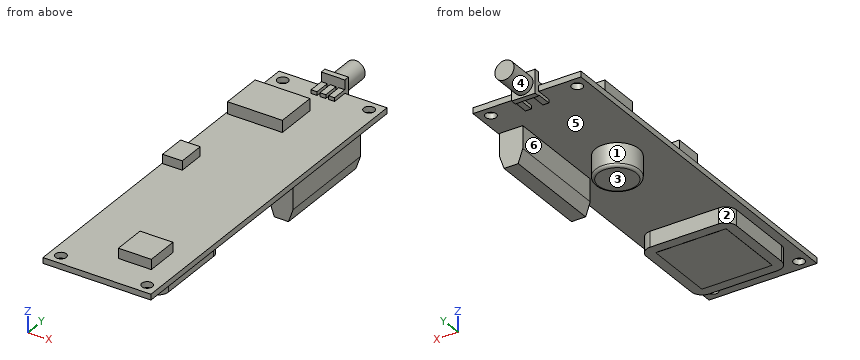
```python
from build123d import *

# Parameters (mm, degrees)
SKETCH3_W            = 1.6002
SKETCH3_H            = 100
BOSS_EXTRUDE1_DEPTH  = 30
SKETCH5_R            = 1.5
SCREW_HOLES_DEPTH    = 13.39
SKETCH7_W            = 6.477
SKETCH7_H            = 28.575
BOSS_EXTRUDE2_DEPTH  = 9.906
CUT_EXTRUDE1_REACH   = 91.18
SKETCH9_R            = 6.0325
BOSS_EXTRUDE3_DEPTH  = 6.35
FILLET1_R            = 0.762
SKETCH10_W           = 25.0698
SKETCH10_H           = 25.0698
BOSS_EXTRUDE4_DEPTH  = 4.318
FILLET2_R            = 3.048
SKETCH11_W           = 19.558
SKETCH11_H           = 19.558
STICKER_DEPTH        = 0.0254
SKETCH12_W           = 15.24
SKETCH12_H           = 11.684
BIG_CHIP_DEPTH       = 3.302
SKETCH13_W           = 9.144
SKETCH13_H           = 9.144
UBLOX_CHIP_DEPTH     = 2.794
SKETCH14_W           = 6.5278
SKETCH14_H           = 6.5278
BOSS_EXTRUDE8_DEPTH  = 1.524
SKETCH15_R           = 2.667
BOSS_EXTRUDE9_DEPTH  = 8.001
SKETCH17_W           = 1.651
SKETCH17_H           = 1.016
BOSS_EXTRUDE10_DEPTH = 4.318
SKETCH18_W           = 1.651
SKETCH18_H           = 0.9652
BOSS_EXTRUDE11_DEPTH = 4.318
SKETCH19_W           = 5.461
SKETCH19_H           = 7.62
USB_CONNECTOR_DEPTH  = 2.54


with BuildPart() as part:
    # Sketch3 → Boss-Extrude1 (new body)
    with BuildSketch(Plane(origin=(0, 0, 0), x_dir=(0, 0, -1), z_dir=(1, 0, 0))):
        with Locations((-0.8001, -50)):
            Rectangle(SKETCH3_W, SKETCH3_H)
    extrude(amount=BOSS_EXTRUDE1_DEPTH)

    # Sketch5 → Screw-Holes (cut)
    with BuildSketch(Plane.XY.offset(1.6002)):
        with Locations((27, -3)):
            Circle(SKETCH5_R)
        with Locations((3, -3)):
            Circle(SKETCH5_R)
        with Locations((3, -97)):
            Circle(SKETCH5_R)
        with Locations((27, -97)):
            Circle(SKETCH5_R)
    extrude(amount=-SCREW_HOLES_DEPTH, mode=Mode.SUBTRACT)

    # Sketch7 → Boss-Extrude2 (add)
    with BuildSketch(Plane(origin=(0, 0, 0), x_dir=(-1, 0, 0), z_dir=(0, 0, -1))):
        with Locations((-26.5075, -25.1079)):
            Rectangle(SKETCH7_W, SKETCH7_H)
    extrude(amount=BOSS_EXTRUDE2_DEPTH)

    # Sketch8 → Cut-Extrude1 (cut, up to next)
    with BuildSketch(Plane(origin=(0, -10.8204, 0), x_dir=(1, 0, 0), z_dir=(0, 1, 0)), mode=Mode.PRIVATE) as cut_extrude1_sk1:
        Polygon((28.476, 9.906), (29.746, 6.223), (29.746, 9.906), align=None)
    cut_extrude1_tool1 = extrude(cut_extrude1_sk1.sketch, amount=-CUT_EXTRUDE1_REACH, mode=Mode.PRIVATE) & part.part
    add(cut_extrude1_tool1.solids().sort_by_distance((29.322667, -10.8204, -8.678333))[0], mode=Mode.SUBTRACT)
    # Sketch8 → Cut-Extrude1 (cut, up to next)
    with BuildSketch(Plane(origin=(0, -10.8204, 0), x_dir=(1, 0, 0), z_dir=(0, 1, 0)), mode=Mode.PRIVATE) as cut_extrude1_sk2:
        Polygon((23.269, 9.906), (23.269, 6.223), (24.539, 9.906), align=None)
    cut_extrude1_tool2 = extrude(cut_extrude1_sk2.sketch, amount=-CUT_EXTRUDE1_REACH, mode=Mode.PRIVATE) & part.part
    add(cut_extrude1_tool2.solids().sort_by_distance((23.692333, -10.8204, -8.678333))[0], mode=Mode.SUBTRACT)

    # Sketch9 → Boss-Extrude3 (add)
    with BuildSketch(Plane(origin=(0, 0, 0), x_dir=(-1, 0, 0), z_dir=(0, 0, -1))):
        with Locations((-12.3825, -34.29)):
            Circle(SKETCH9_R)
    extrude(amount=BOSS_EXTRUDE3_DEPTH)

    # Fillet1
    fillet1_edges = [part.edges().sort_by_distance(p)[0] for p in [
        (18.415, -34.29, -6.35),
    ]]
    fillet(fillet1_edges, radius=FILLET1_R)

    # Sketch10 → Boss-Extrude4 (add)
    with BuildSketch(Plane(origin=(0, 0, 0), x_dir=(-1, 0, 0), z_dir=(0, 0, -1))):
        with Locations((-15, -79.2101)):
            Rectangle(SKETCH10_W, SKETCH10_H)
    extrude(amount=BOSS_EXTRUDE4_DEPTH)

    # Fillet2
    fillet2_edges = [part.edges().sort_by_distance(p)[0] for p in [
        (2.4651, -91.745, -2.159),
        (2.4651, -66.6752, -2.159),
        (27.5349, -66.6752, -2.159),
        (27.5349, -91.745, -2.159),
    ]]
    fillet(fillet2_edges, radius=FILLET2_R)

    # Sketch11 → Sticker (add)
    with BuildSketch(Plane(origin=(0, 0, -4.318), x_dir=(-1, 0, 0), z_dir=(0, 0, -1))):
        with Locations((-15, -79.2101)):
            Rectangle(SKETCH11_W, SKETCH11_H)
    extrude(amount=STICKER_DEPTH)

    # Sketch12 → Big chip (add)
    with BuildSketch(Plane.XY.offset(1.6002)):
        with Locations((8.128, -16.764)):
            Rectangle(SKETCH12_W, SKETCH12_H)
    extrude(amount=BIG_CHIP_DEPTH)

    # Sketch13 → ublox chip (add)
    with BuildSketch(Plane.XY.offset(1.6002)):
        with Locations((19.459, -86.157)):
            Rectangle(SKETCH13_W, SKETCH13_H)
    extrude(amount=UBLOX_CHIP_DEPTH)

    # Sketch14 → Boss-Extrude8 (add)
    with BuildSketch(Plane(origin=(0, 0, 0), x_dir=(1, 0, 0), z_dir=(0, 1, 0))):
        with Locations((15, -1.9939)):
            Rectangle(SKETCH14_W, SKETCH14_H)
    extrude(amount=BOSS_EXTRUDE8_DEPTH)

    # Sketch15 → Boss-Extrude9 (add)
    with BuildSketch(Plane(origin=(0, 1.524, 0), x_dir=(1, 0, 0), z_dir=(0, 1, 0))):
        with Locations((15, -1.9939)):
            Circle(SKETCH15_R)
    extrude(amount=BOSS_EXTRUDE9_DEPTH)

    # Sketch17 → Boss-Extrude10 (add)
    with BuildSketch(Plane.XZ):
        with Locations((15, 2.1082)):
            Rectangle(SKETCH17_W, SKETCH17_H)
        with Locations((12.5616, 2.1082)):
            Rectangle(SKETCH17_W, SKETCH17_H)
        with Locations((17.4384, 2.1082)):
            Rectangle(SKETCH17_W, SKETCH17_H)
    extrude(amount=BOSS_EXTRUDE10_DEPTH)

    # Sketch18 → Boss-Extrude11 (add)
    with BuildSketch(Plane.XZ):
        with Locations((12.5616, -0.4826)):
            Rectangle(SKETCH18_W, SKETCH18_H)
        with Locations((17.4384, -0.4826)):
            Rectangle(SKETCH18_W, SKETCH18_H)
    extrude(amount=BOSS_EXTRUDE11_DEPTH)

    # Sketch19 → USB connector (add)
    with BuildSketch(Plane.XY.offset(1.6002)):
        with Locations((2.8575, -45.72)):
            Rectangle(SKETCH19_W, SKETCH19_H)
    extrude(amount=USB_CONNECTOR_DEPTH)


solid = part.part
```
Could you check a few things on this model? Use its own coordinates, in mm. Face numbers are marked on the shaded views. A direction names the side the tool comes from. Give positions to 0.01 mm unless a question says otherwise; leave off trailing zeros. Loops run counter-clockwise (first coordinate to the right, second up) from the corner with the lowest first, then second, coordinate; pieces in that order, holes last. Notation, with made-up numbers: (30.25, 52) - (75.25, 52) arc R29 ccw to (75.25, 73) - close; hole circle Ø1 at (86.5, 20.25). An arc over 180 degrees is marked (long way). Answer in a Markdown table with one row per item. Add a question column.
Q1. Which directions (+Z, -Z, +X, -X, +Y, -Y) give clear straight access to the entire face, cutting with the end or side of a thin tool? Please do the marked faces 4, 5 and 6.
Q2. If we section it at B-B (z = -2.5): State how many separate pieces and enclosed holes the cut face has, plus the area to 3 significant figures.
Q3. If we section it at A-A (y = -97): List the corners of the cut face in (x, z) for me, plus the area to 3 significant figures.
Q4. We'd pull the mould along X, two halves only. Please class the marked faces 1, 2 and 3: +X half, -X half, draft (parallel to the pull), parting line (faces both ways), or undercut.
Q5. For pin 1 (5 mm diameter, centred on y = -30.5, z = -3, fed in from -X); pin 2 (1.5 mm diameter, centred on y = -14.5, z = -1, fed in from -X); pin 3 (2.5 mm diameter, centred on y = -14, z = 3, fed in from -X); pin 4 (1 mm diameter, centred on y = -40, z = 2.5, fed in from +X), each with a flat end and sliding along its axis, tell me the tip position at first contact or that it passes through.
Q6. If we section it at D-D (y = -20.5): List the corners of the cut face in (x, z) for me, plus the area to 3 significant figures.
Q7. If we section it at C-C (y = -34.29): List the corners of the cut face in (x, z) for me (3 decimals), plus the area to 3 significant figures.
Q8. Please list where these lines run through material, in increasing order: L1, parallel to Y at x = 27, z = 0.45; L2, parallel to X at y = -97, z = 0.85; L3, parallel to X at y = -13, z = -6.25. Write a range as from..to.
The answers:
| question | item | result |
|---|---|---|
| 1 | face 4 | +Y |
| 1 | face 5 | -Z |
| 1 | face 6 | -Z, +Y |
| 2 | separate pieces | 3 |
| 2 | enclosed holes | 0 |
| 2 | area | 920 mm^2 |
| 3 | outline | (0, 0) - (1.5, 0) - (1.5, 1.6) - (0, 1.6) - close; (4.5, 0) - (25.5, 0) - (25.5, 1.6) - (4.5, 1.6) - close; (28.5, 0) - (30, 0) - (30, 1.6) - (28.5, 1.6) - close |
| 3 | area | 38.4 mm^2 |
| 4 | face 1 | undercut |
| 4 | face 2 | -X half |
| 4 | face 3 | draft |
| 5 | pin 1 | stops at x = 6.49 |
| 5 | pin 2 | stops at x = 23.27 |
| 5 | pin 3 | stops at x = 0.51 |
| 5 | pin 4 | passes through |
| 6 | outline | (0, 0) - (23.27, 0) - (23.27, -6.22) - (24.54, -9.91) - (28.48, -9.91) - (29.75, -6.22) - (29.75, 0) - (30, 0) - (30, 1.6) - (15.75, 1.6) - (15.75, 4.9) - (0.51, 4.9) - (0.51, 1.6) - (0, 1.6) - close |
| 6 | area | 158 mm^2 |
| 7 | outline | (0, 0) - (6.35, 0) - (6.35, -5.588) arc R0.762 ccw to (7.112, -6.35) - (17.653, -6.35) arc R0.762 ccw to (18.415, -5.588) - (18.415, 0) - (23.269, 0) - (23.269, -6.223) - (24.539, -9.906) - (28.476, -9.906) - (29.746, -6.223) - (29.746, 0) - (30, 0) - (30, 1.6) - (0, 1.6) - close |
| 7 | area | 184 mm^2 |
| 8 | L1 | y = -100..-98.5, -95.5..-4.5, -1.5..0 |
| 8 | L2 | x = 0..1.5, 4.5..25.5, 28.5..30 |
| 8 | L3 | x = 23.28..29.74 |
